Part model, mm, in its own coordinate system. Coordinates: 2 decimals unless noted, no trailing zeros. Loops run counter-clockwise (first coordinate to the right, second up) from the corner with the lowest first, then second, coordinate; pieces in that order, holes last. Notation, with made-up numbers: (25, -36) - (53, -36) arc R18 ccw to (53, -6) - close; hole circle Ø6 at (-21, 42). An arc over 180 degrees is marked (long way). Use a Markdown table: item, result. Add a question column.
1) Band-saw the part on A-A (x = 44). Give the cut face in (y, z).
2) Pull direction X, two halves, no side cores. Call faces 1 (the face through (24, 0, 1)), 2 (the face through (0, 12, 1)), 3 (the face through (5.13, 21.77, 1.01)): +X half, -X half, draft (parallel to the pull), parting line (faces both ways), or undercut.
3) Band-saw the part on B-B (y = 12). Give the cut face in (x, z).
4) Band-saw the part on C-C (z = 1.55). Give the number of separate pieces and of enclosed holes in the cut face, plus the area to 3 significant figures.
5) Band-saw the part on D-D (x = 36.5). Give the cut face in (y, z), plus the area to 3 significant figures.
6) Probe probe 1 along Y at (x, z) = (36, 0.7); probe 2 along Y at (x, z) = (4.5, 1.3). List the from-to ranges inside material, lowest first. Write a range as [from, to].
from build123d import *

# Parameters (mm, degrees)
ESQUISSE1_W                     = 48
ESQUISSE1_H                     = 24
BOSS_EXTRU_1_DEPTH              = 2
ESQUISSE2_R                     = 2.1
ENL_V_MAT_EXTRU_1_DEPTH         = 54.702886328
R_P_TITION_LIN_AIRE1_COUNT      = 3
R_P_TITION_LIN_AIRE1_PITCH      = 8
R_P_TITION_LIN_AIRE1_COUNT_DIR2 = 6
R_P_TITION_LIN_AIRE1_PITCH_DIR2 = 8


with BuildPart() as part:
    # Esquisse1 → Boss.-Extru.1 (new body)
    with BuildSketch(Plane.XY):
        with Locations((24, 12)):
            Rectangle(ESQUISSE1_W, ESQUISSE1_H)
    extrude(amount=BOSS_EXTRU_1_DEPTH)

    # Esquisse2 → Enlèv. mat.-Extru.1 (cut, through all)
    with BuildSketch(Plane.XY.offset(2)):
        with Locations((4, 20)):
            Circle(ESQUISSE2_R)
    enl_v_mat_extru_1 = extrude(amount=-ENL_V_MAT_EXTRU_1_DEPTH, mode=Mode.SUBTRACT)

    # Répétition linéaire1: Enl_v. mat.-Extru.1 3 × 6
    with Locations(*[(j * R_P_TITION_LIN_AIRE1_PITCH_DIR2, -i * R_P_TITION_LIN_AIRE1_PITCH, 0) for i in range(R_P_TITION_LIN_AIRE1_COUNT) for j in range(R_P_TITION_LIN_AIRE1_COUNT_DIR2) if (i, j) != (0, 0)]):
        add(enl_v_mat_extru_1, mode=Mode.SUBTRACT)


solid = part.part
Answer block:
| question | item | result |
|---|---|---|
| 1 | outline | (0, 0) - (1.9, 0) - (1.9, 2) - (0, 2) - close; (6.1, 0) - (9.9, 0) - (9.9, 2) - (6.1, 2) - close; (14.1, 0) - (17.9, 0) - (17.9, 2) - (14.1, 2) - close; (22.1, 0) - (24, 0) - (24, 2) - (22.1, 2) - close |
| 2 | face 1 | draft |
| 2 | face 2 | -X half |
| 2 | face 3 | undercut |
| 3 | outline | (0, 0) - (1.9, 0) - (1.9, 2) - (0, 2) - close; (6.1, 0) - (9.9, 0) - (9.9, 2) - (6.1, 2) - close; (14.1, 0) - (17.9, 0) - (17.9, 2) - (14.1, 2) - close; (22.1, 0) - (25.9, 0) - (25.9, 2) - (22.1, 2) - close; (30.1, 0) - (33.9, 0) - (33.9, 2) - (30.1, 2) - close; (38.1, 0) - (41.9, 0) - (41.9, 2) - (38.1, 2) - close; (46.1, 0) - (48, 0) - (48, 2) - (46.1, 2) - close |
| 4 | separate pieces | 1 |
| 4 | enclosed holes | 18 |
| 4 | area | 903 mm2 |
| 5 | outline | (0, 0) - (1.96, 0) - (1.96, 2) - (0, 2) - close; (6.04, 0) - (9.96, 0) - (9.96, 2) - (6.04, 2) - close; (14.04, 0) - (17.96, 0) - (17.96, 2) - (14.04, 2) - close; (22.04, 0) - (24, 0) - (24, 2) - (22.04, 2) - close |
| 5 | area | 23.5 mm2 |
| 6 | probe 1 | [0, 1.9], [6.1, 9.9], [14.1, 17.9], [22.1, 24] |
| 6 | probe 2 | [0, 1.96], [6.04, 9.96], [14.04, 17.96], [22.04, 24] |
